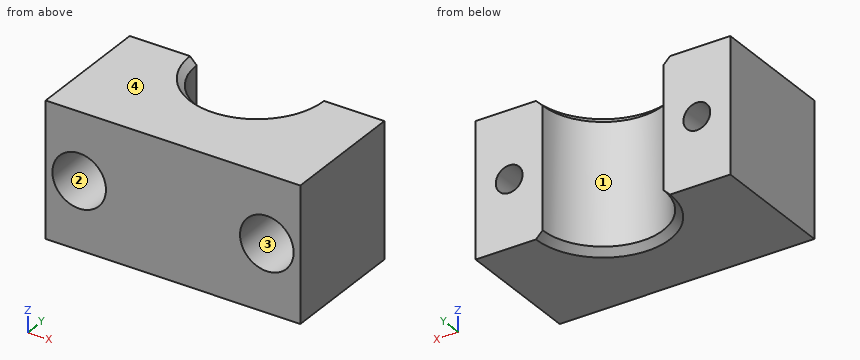
from build123d import *

# Parameters (mm, degrees)
F1_DEPTH = 20
F2_R     = 2
F3_DEPTH = 19.001
F4_R     = 4
F5_DEPTH = 14
F6_SIZE  = 1


with BuildPart() as f1:
    # F0 (on Top) → F1 (new body)
    with BuildSketch(Plane.XY):
        with BuildLine():
            Line((-9, 9.5), (-19, 9.5))
            Line((-19, 9.5), (-19, -9.5))
            Line((-19, -9.5), (19, -9.5))
            Line((19, -9.5), (19, 9.5))
            Line((19, 9.5), (9, 9.5))
            ThreePointArc((9, 9.5), (0, 0.5), (-9, 9.5))
        make_face()
    extrude(amount=F1_DEPTH)

    # F2 (on face) → F3 (cut, through all)
    with BuildSketch(Plane(origin=(0, 9.5, 0), x_dir=(-1, 0, 0), z_dir=(0, 1, 0))):
        with Locations((-14, 10)):
            Circle(F2_R)
        with Locations((14, 10)):
            Circle(F2_R)
    extrude(amount=-F3_DEPTH, mode=Mode.SUBTRACT)

    # F4 (on face) → F5 (cut)
    with BuildSketch(Plane.XZ.offset(9.5)):
        with Locations((-14, 10)):
            Circle(F4_R)
        with Locations((14, 10)):
            Circle(F4_R)
    extrude(amount=-F5_DEPTH, mode=Mode.SUBTRACT)

    # F6
    f6_edges = [f1.edges().sort_by_distance(p)[0] for p in [
        (0, 0.5, 0),
        (0, 0.5, 20),
    ]]
    chamfer(f6_edges, length=F6_SIZE)


solid = f1.part
Check sheet for the modelled part. Datum: model origin and axes. Units: mm. Face numbers are marked on the shaded views. Round coordinates to 2 decimals unless told otherwise and drop trailing zeros. Loops run counter-clockwise (first coordinate to the right, second up) from the corner with the lowest first, then second, coordinate; pieces in that order, holes last. Notation, with made-up numbers: (89.25, 35) -> (138.25, 35) arc R26 cw to (138.25, 66) -> close; hole circle Ø11 at (18.5, 69.5). An arc over 180 degrees is marked (long way). Put each result on its own line as item: value. Start each with the question number.
1. Gauge pin test, flat ends, axial feed: pin 1 (7 mm diameter, centred on x = -14, z = 10, fed in from +Y); pin 2 (2.5 mm diameter, centred on x = -14, z = 12, fed in from -Y); pin 3 (1.5 mm diameter, centred on x = -6.5, z = 7.5, fed in from +Y). Record the tip position at first contact, or that the pin passes through.
2. Section check D-D (z = 3.5). Enter the section's corners in (x, y), plus the area to 3 significant figures.
3. Section check A-A (z = 10). Enter the section's corners in (x, y), plus the area to 3 significant figures.
4. Section check C-C (y = -2). Enter the section's corners in (x, z), plus the area to 3 significant figures.
5. Draft check along Z on the marked faces 1, 2, 3 and 4. Enter one of: +Z half, -Z half, draft (parallel to the pull), parting line (faces both ways), or undercut.
6. Scan lines: probe 1 along X at (y, z) = (-3.25, 9.75); probe 2 along Z at (x, y) = (14, -2.25); probe 3 along Z at (x, y) = (14, 8.4). Record each from-to range of solid material in increasing order.
7. Section check B-B (x = 14). Enter the section's corners in (y, z).
Findings:
1. pin 1: stops at y = 9.5
1. pin 2: stops at y = 4.5
1. pin 3: stops at y = 4.17
2. outline: (-19, -9.5) -> (19, -9.5) -> (19, 9.5) -> (9, 9.5) arc R9 cw to (-9, 9.5) -> (-19, 9.5) -> close
2. area: 595 mm^2
3. outline: (-19, -9.5) -> (-18, -9.5) -> (-18, 4.5) -> (-16, 4.5) -> (-16, 9.5) -> (-19, 9.5) -> close; (-12, 4.5) -> (-10, 4.5) -> (-10, -9.5) -> (10, -9.5) -> (10, 4.5) -> (12, 4.5) -> (12, 9.5) -> (9, 9.5) arc R9 cw to (-9, 9.5) -> (-12, 9.5) -> close; (16, 4.5) -> (18, 4.5) -> (18, -9.5) -> (19, -9.5) -> (19, 9.5) -> (16, 9.5) -> close
3. area: 331 mm^2
4. outline: (-19, 0) -> (19, 0) -> (19, 20) -> (-19, 20) -> close; hole circle Ø8 at (-14, 10); hole circle Ø8 at (14, 10)
4. area: 659 mm^2
5. face 1: draft
5. face 2: undercut
5. face 3: undercut
5. face 4: +Z half
6. probe 1: x = -19 to -17.99, -10.01 to 10.01, 17.99 to 19
6. probe 2: z = 0 to 6, 14 to 20
6. probe 3: z = 0 to 8, 12 to 20
7. outline: (-9.5, 0) -> (9.5, 0) -> (9.5, 8) -> (4.5, 8) -> (4.5, 6) -> (-9.5, 6) -> close; (-9.5, 14) -> (4.5, 14) -> (4.5, 12) -> (9.5, 12) -> (9.5, 20) -> (-9.5, 20) -> close
